CAD build for the part. Positions are in the model's coordinates, mm. A direction names the side the tool comes from. Give positions to 0.01 mm unless a question says otherwise; leave off trailing zeros. Order: outer loops, then holes, each group sorted by start corner. A loop starts at its lowest first (then second) coordinate and runs counter-clockwise, first axis right, second up.
Item 1: Wall check: L1, parallel to Z at x = -10, y = 5.75; L2, parallel to X at y = -2.75, z = 10.75; L3, parallel to X at y = -0.75, z = 7.5. Give the ranges that are in metal, low to high.
Item 2: Band-saw the part on B-B on x = 10. Give the cut face in (y, z) (3 decimals), plus the area to 3 significant figures.
Item 3: Flat gauge pins, fed straight in: P1, Ø1.5, axis at x = 4.5, y = 2.5, coming from the -Z side; P2, Ø2.5, axis at x = 0, y = 0, coming from the +Z side; P3, Ø5, axis at x = -10, z = -10.75, coming from the -Y side (3 decimals); P4, Ø1.5, axis at x = 6.5, y = -1, coming from the +Z side. Where does each tip first touch, or does it go through?
Item 4: Two-plate mould, pull along Z, no slides. Class faces 5 (the cylindrical face through (0.867, 3.905, -16.226)), 6 (the flat face through (-3, 4, 14.5)), 7 (the cylindrical face through (-11.19, 0.09, 11.66)): released by +Z, released by -Z, zero draft, split by the parting line, or undercut.
Item 5: Band-saw the part on C-C on z = 10.75. Give the cut face in (x, y) (3 decimals), plus the area to 3 significant figures.
Item 6: Band-saw the part on D-D on z = 3.5. Give the cut face in (x, y) (3 decimals).
Item 7: Which spindle directions (+Z, -Z, +X, -X, +Y, -Y) get a long thin tool onto all of the face, cutting with end or side? Do faces 1 (the flat face through (7.25, 0, 0)), 2 (the cylindrical face through (-10, 0, -3)), 3 (the cylindrical face through (0, 3, 17)), 4 (the flat face through (9, -6.375, 0)). Say none if no direction does.
Item 8: Band-saw the part on A-A on x = -10. Give the cut face in (y, z) (3 decimals), plus the area to 3 significant figures.
Autodesk Inventor part; units mm, degrees
ref_plane "YZ Plane" through (0, 0, 0) normal (1, 0, 0) x (0, 1, 0)
ref_plane "XZ Plane" through (0, 0, 0) normal (0, 1, 0) x (-1, 0, 0)
ref_plane "XY Plane" through (0, 0, 0) normal (0, 0, 1) x (1, 0, 0)
sketch "Sketch1" plane through (0, 0, 0) normal (0, 1, 0) x (-1, 0, 0)
  line L0 (12.75, -14.5) -> (-12.75, -14.5)
  line L1 (-12.75, -14.5) -> (-12.75, 14.5)
  line L2 (-12.75, 14.5) -> (12.75, 14.5)
  line L3 (12.75, 14.5) -> (12.75, -14.5)
  line L4 (12.75, -14.5) -> (-12.75, 14.5) construction
  line L5 (-12.75, -14.5) -> (12.75, 14.5) construction
  point P0 (0, 0)
  dimension "d0" = 25.5
  dimension "d1" = 29
extrude "Extrusion1" add sketch "Sketch1" along normal mid plane 12.75
sketch "Sketch2" plane through (0, 6.375, 0) normal (0, 1, 0) x (1, 0, 0)
  line L0 (-7.25, 9.5) -> (7.25, 9.5)
  line L1 (7.25, 9.5) -> (7.25, -9.5)
  line L2 (7.25, -9.5) -> (-7.25, -9.5)
  line L3 (-7.25, -9.5) -> (-7.25, 9.5)
  line L4 (-7.25, 9.5) -> (7.25, -9.5) construction
  line L5 (7.25, 9.5) -> (-7.25, -9.5) construction
  point P0 (0, 0)
  dimension "d4" = 14.5
  dimension "d5" = 19
extrude "Extrusion2" cut sketch "Sketch2" against normal blind 12.75
sketch "Sketch3" plane through (0, 6.375, 0) normal (0, 1, 0) x (1, 0, 0)
  circle A0 centre (10, 10.75) radius 1.5
  line L0 (12.75, 14.5) -> (-12.75, 14.5)
  line L1 (12.75, -14.5) -> (12.75, 14.5)
  circle A1 centre (-10, 10.75) radius 1.5
  circle A2 centre (10, -10.75) radius 1.5
  circle A3 centre (-10, -10.75) radius 1.5
  point P0 (0, 0)
  dimension "d8" = 3
  dimension "d9" = 3.75
  dimension "d10" = 2.75
  dimension "d13" = 20
  dimension "d16" = 21.5
sketch "Sketch4" plane through (-12.75, 6.375, 14.5) normal (0, 0, 1) x (1, 0, 0)
  circle A0 centre (12.75, -6.375) radius 4.75
  dimension "d19" = 9.5
extrude "Extrusion3" add sketch "Sketch4" along normal blind 5.5
extrude "Extrusion6" cut sketch "Sketch3" against normal through all
sketch "Sketch7" plane through (12.75, 6.375, -14.5) normal (0, 0, -1) x (-1, 0, 0)
  circle A0 centre (12.75, -6.375) radius 1.2632
  circle A1 centre (12.75, -6.375) radius 4
  point P0 (12.75, -6.375)
  dimension "d32" = 8
extrude "Extrusion7" add sketch "Sketch7" along normal blind 7.5 contours A0 | A1
sketch "Sketch8" plane through (-12.75, -6.375, 14.5) normal (-1, 0, 0) x (0, 0, 1)
  circle A0 centre (-14.5, 6.375) radius 3
  dimension "d35" = 6
hole "Hole1" at (-12.75, 0, 0) direction (1, 0, 0) diameter 6 depth 8 tip angle 118
thread "Thread2"
fillet "Fillet1" [suppressed]
sketch "Sketch10" plane through (0, 0, 20) normal (0, 0, 1) x (1, 0, 0)
  circle A0 centre (0, 0) radius 1.5
  point P0 (0, 0)
hole "Hole2" at (0, 0, 20) direction (0, 0, -1) diameter 6 depth 6 tip angle 118
sketch "Sketch11" plane through (7.25, 6.375, 9.5) normal (0, 0, -1) x (-1, 0, 0)
  circle A0 centre (7.25, -6.375) radius 1.5
hole "Hole3" at (0, 0, 9.5) direction (0, 0, 1) diameter 3 end through all
thread "Thread3"
fillet "Fillet2" radius 4 1 edges at (4, 0, -22)
sketch "Sketch12" plane through (-7.25, 6.375, -9.5) normal (0, 0, 1) x (1, 0, 0)
  point P0 (7.25, -6.375)
  point P1 (7.25, -6.375)
sketch "Sketch13" plane through (0, 0, 0) normal (0, 1, 0) x (-1, 0, 0)
  line L0 (-4, -18) -> (4, -18)
  line L1 (4.75, 20) -> (-4.75, 20)
  point P0 (0, 0)
  point P1 (0, -18)
  dimension "d67" = 38
hole "Hole4" at (0, 0, -9.5) direction (0, 0, -1) diameter 3 depth 8.5 tip angle 118
properties material "Iron, Cast"
The answers:
1. L1: z = -14.5 to -12.25, -9.25 to 9.25, 12.25 to 14.5
1. L2: x = -12.75 to -11.5, -8.5 to 8.5, 11.5 to 12.75
1. L3: x = -12.75 to -7.25, 7.25 to 12.75
2. outline: (-6.375, -14.5) - (6.375, -14.5) - (6.375, -12.25) - (-6.375, -12.25) - close; (-6.375, -9.25) - (6.375, -9.25) - (6.375, 9.25) - (-6.375, 9.25) - close; (-6.375, 12.25) - (6.375, 12.25) - (6.375, 14.5) - (-6.375, 14.5) - close
2. area: 293 mm2
3. P1: stops at z = -14.5
3. P2: stops at z = -18.15
3. P3: stops at y = -6.375
3. P4: stops at z = 14.5
4. face 5: zero draft
4. face 6: released by +Z
4. face 7: undercut
5. outline: (-12.75, -6.375) - (-11.5, -6.375) - (-11.5, 6.375) - (-12.75, 6.375) - close; (-8.5, -6.375) - (8.5, -6.375) - (8.5, 6.375) - (-8.5, 6.375) - close; (11.5, -6.375) - (12.75, -6.375) - (12.75, 6.375) - (11.5, 6.375) - close; hole circle Ø3 at (0, 0)
5. area: 242 mm2
6. outline: (-12.75, -6.375) - (-7.25, -6.375) - (-7.25, 6.375) - (-12.75, 6.375) - close; (7.25, -6.375) - (12.75, -6.375) - (12.75, 6.375) - (7.25, 6.375) - close
7. face 1: +Y, -Y
7. face 2: -X
7. face 3: +Z
7. face 4: +Z, -Z, +X, -X, -Y
8. outline: (-6.375, -14.5) - (6.375, -14.5) - (6.375, -12.25) - (-6.375, -12.25) - close; (-6.375, -9.25) - (6.375, -9.25) - (6.375, 9.25) - (-6.375, 9.25) - close; (-6.375, 12.25) - (6.375, 12.25) - (6.375, 14.5) - (-6.375, 14.5) - close; hole circle Ø6 at (0, 0)
8. area: 265 mm2
